```python
from build123d import *

# Parameters (mm, degrees)
F1_DEPTH = 63.5
F2_DEPTH = 25.4
F3_DEPTH = 7.9375
F5_R     = 6.35


with BuildPart() as f1:
    # F0 (on Front) → F1 (new body, symmetric)
    with BuildSketch(Plane.XZ):
        Polygon((-41.275, 9.525), (-41.275, -9.525), (41.275, -9.525), (41.275, 9.525), (22.225, 9.525), align=None)
    extrude(amount=F1_DEPTH, both=True)

    # F0 (on Front) → F2 (join, symmetric)
    with BuildSketch(Plane.XZ):
        Polygon((79.7655956935, 61.9252), (60.325, 61.9252), (60.325, 42.8752), (79.5641856105, 42.8752), align=None)
        with BuildLine():
            Line((22.225, 9.525), (41.275, 9.525))
            Line((41.275, 9.525), (41.275, 27.0002))
            ThreePointArc((41.275, 27.0002), (45.9246798487, 38.2255201513), (57.15, 42.8752))
            Line((57.15, 42.8752), (60.325, 42.8752))
            Line((60.325, 42.8752), (60.325, 61.9252))
            Line((60.325, 61.9252), (57.15, 61.9252))
            add(Edge.make_bspline(
                [(55.693596433, 61.8948201247), (56.1824633376, 61.9077141439), (56.6679863057, 61.9178418733), (57.15, 61.9252)],
                knots=[110.0991470384, 110.0991470384, 110.0991470384, 110.0991470384, 111.5045361635, 111.5045361635, 111.5045361635, 111.5045361635], degree=3))
            ThreePointArc((55.693596433, 61.8948201247), (31.944638273, 51.1755048628), (22.225, 27.0002))
            Line((22.225, 27.0002), (22.225, 9.525))
        make_face()
    extrude(amount=F2_DEPTH, both=True)

    # F0 (on Front) → F3 (join, symmetric)
    with BuildSketch(Plane.XZ):
        with BuildLine():
            add(Edge.make_bspline(
                [(-41.275, 9.525), (-41.4253577481, 42.8971199806), (17.395428152, 60.8846938277), (55.693596433, 61.8948201247)],
                knots=[0, 0, 0, 0, 110.0991470384, 110.0991470384, 110.0991470384, 110.0991470384], degree=3))
            Line((-41.275, 9.525), (22.225, 9.525))
            Line((22.225, 9.525), (22.225, 27.0002))
            ThreePointArc((22.225, 27.0002), (31.944638273, 51.1755048628), (55.693596433, 61.8948201247))
        make_face()
    extrude(amount=F3_DEPTH, both=True)

    # F0 (on Front) → F4 (revolve)
    with BuildSketch(Plane.XZ):
        Polygon((79.8158139409, 66.675), (79.7655956935, 61.9252), (79.5641856105, 42.8752), (79.5136988163, 38.1), (111.125, 38.1), (111.125, 66.675), align=None)
    revolve(axis=Axis((79.6647563786, 0, 52.3875), (0.0105721169, 0, 0.9999441136)))

    # F5
    f5_edges = [f1.edges().sort_by_distance(p)[0] for p in [
        (41.275, -63.5, 0),
        (-41.275, -63.5, 0),
        (-41.275, 63.5, 0),
        (41.275, 63.5, 0),
    ]]
    fillet(f5_edges, radius=F5_R)


solid = f1.part
```
For this review, take the finished solid that the model builds, in its own axes (mm). A direction names the side the tool comes from. Coordinates: 2 decimals unless noted, no trailing zeros. Loops run counter-clockwise (first coordinate to the right, second up) from the corner with the lowest first, then second, coordinate; pieces in that order, holes last. Notation, with made-up numbers: (-24, -29) -> (-5, -29) arc R12 ccw to (-5, -24) -> close; hole circle Ø2 at (25, 17). An arc over 180 degrees is marked (long way). Return JSON: item names as keys, results as strings. Group by question number.
(1) To check wall thickness, follow L1, parallel to X at y = -55, z = -1.5 (3 decimals); L2, parallel to Z at x = -21.5, y = 43.5 (3 decimals); L3, parallel to Y at x = 43.5, z = 48. State the ranges of each line that lie inside material, in increasing order.
(2) Consider section B-B, the plane y = 44. Give the boundary of the cut face in (x, z) (3 decimals), plus the area to 3 significant figures.
(3) Mouldability with a two-part tool opening along X and no side actions: class faces 1 (the cylindrical face through (32.2, -16.79, 51.44)), 2 (the conical face through (77.54, 0.09, 38.14)), 3 (the flat face through (-5, 7.938, 30)), 4 (the cylindrical face through (39.464, 61.59, 0.133)) as pulls with the +X half, pulls with the -X half, needs draft (parallel to the pull), parting line crosses it, or undercut.
(4) Tool access review of faces 5 (the flat face through (22.225, -17, 18)), 6 (the flat face through (41.275, -1, 4)), 7 (the flat face through (58, 24, 61.925)): name each direction out of +Z, -Z, +X, -X, +Y, -Y from which nothing blocks a thin tool from reaching the whole face with its end or side.
(5) For pin 1 Ø8 at (x, y) = (48.5, 27.5) entering from +Z; pin 2 Ø5 at (x, y) = (-12.5, -33.5) entering from +Z (3 decimals); pin 3 Ø4 at (x, y) = (59, 24.5) entering from +Z, all flat-tipped, find the tip position at first contact; note any pin that passes through.
Results below:
{
 "1": {"L1": "x = -41.275 to 41.275", "L2": "z = -9.525 to 9.525", "L3": "y = -25.4 to 25.4"},
 "2": {"outline": "(-41.275, -9.525) -> (41.275, -9.525) -> (41.275, 9.525) -> (-41.275, 9.525) -> close", "area": "1,570 mm2"},
 "3": {"face 1": "pulls with the -X half", "face 2": "undercut", "face 3": "needs draft", "face 4": "pulls with the +X half"},
 "4": {"face 5": "+Z, -X, -Y", "face 6": "-Z, +X, +Y, -Y", "face 7": "+Z, -X, +Y"},
 "5": {"pin 1": "stops at z = 61.53", "pin 2": "stops at z = 9.525", "pin 3": "stops at z = 67.23"}
}
